Model file for the job. Use its own axes, mm. Face numbers are marked on the shaded views. A direction names the side the tool comes from. Round coordinates to 2 decimals unless told otherwise and drop trailing zeros. Loops run counter-clockwise (first coordinate to the right, second up) from the corner with the lowest first, then second, coordinate; pieces in that order, holes last. Notation, with made-up numbers: M -15,-28.75 L 18,-28.75 A27 cw 18,3.25 Z; hole C -24.5,43.25 d10. An arc over 180 degrees is marked long. Answer in a Markdown table with one row per item.
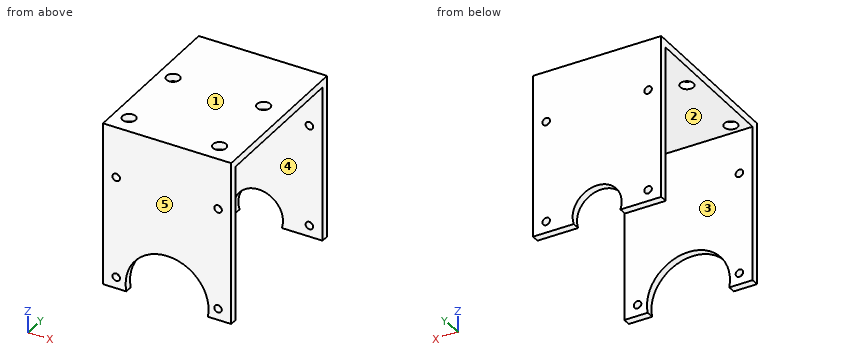
Autodesk Inventor part; units mm, degrees
ref_plane "YZ Plane" through (0, 0, 0) normal (1, 0, 0) x (0, 1, 0)
ref_plane "XZ Plane" through (0, 0, 0) normal (0, 1, 0) x (-1, 0, 0)
ref_plane "XY Plane" through (0, 0, 0) normal (0, 0, 1) x (1, 0, 0)
sketch "スケッチ1" plane through (0, 0, 0) normal (0, 1, 0) x (-1, 0, 0)
  line L0 (0, 0) -> (-34, 0)
  line L1 (-34, 0) -> (-34, -43.5)
  line L2 (-34, -43.5) -> (0, -43.5)
  line L3 (0, -43.5) -> (0, 0)
  dimension "d0" = 43.5
  dimension "d1" = 34
extrude "押し出し1" add sketch "スケッチ1" along normal blind 43.5
sketch "スケッチ2" plane through (34, 0, 0) normal (1, 0, 0) x (0, 0, -1)
  line L0 (2, 41.5) -> (52, 41.5)
  line L1 (52, 41.5) -> (52, 2)
  line L2 (52, 2) -> (2, 2)
  line L3 (2, 2) -> (2, 41.5)
  line L4 (0, 43.5) -> (43.5, 43.5)
  line L5 (0, 0) -> (0, 43.5)
  dimension "d4" = 2
  dimension "d5" = 2
  dimension "d6" = 39.5
  dimension "d7" = 50
extrude "押し出し2" cut sketch "スケッチ2" against normal blind 43.5
sketch "スケッチ3" plane through (0, 0, 0) normal (0, -1, 0) x (1, 0, 0)
  circle A0 centre (17, -41.5) radius 11
  line L0 (34, -43.5) -> (0, -43.5)
  line L1 (0, -43.5) -> (0, 0)
  point P0 (6.1833, -43.5)
  point P1 (27.8167, -43.5)
  dimension "d10" = 22
  dimension "d11" = 2
  dimension "d12" = 17
extrude "押し出し3" cut sketch "スケッチ3" against normal blind 2 contours A0 L0 picked at (20.7405, -37.2254)
sketch "スケッチ4" plane through (0, 43.5, 0) normal (0, 1, 0) x (1, 0, 0)
  circle A0 centre (17, 41.5) radius 6.5
  line L0 (34, 43.5) -> (0, 43.5)
  line L1 (0, 43.5) -> (0, 0)
  point P0 (23.1847, 43.5)
  point P1 (10.8153, 43.5)
  point P2 (0, 35.0774)
  dimension "d15" = 13
  dimension "d16" = 2
  dimension "d17" = 17
extrude "押し出し4" cut sketch "スケッチ4" against normal blind 2
sketch "スケッチ5" plane through (0, 43.5, 0) normal (0, 1, 0) x (1, 0, 0)
  line L0 (0, 0) -> (34, 0)
  line L1 (0, 43.5) -> (0, 0)
  line L2 (34, 0) -> (34, 43.5)
  point P0 (3.5, 13.5)
  point P1 (3.5, 40.5)
  point P2 (30.5, 40.5)
  point P3 (30.5, 13.5)
  dimension "d20" = 13.5
  dimension "d21" = 3.5
  dimension "d22" = 27
  dimension "d23" = 3.5
  dimension "d48" = 3.5
hole "穴1" at (3.5, 43.5, -13.5) at (3.5, 43.5, -40.5) at (30.5, 43.5, -40.5) at (30.5, 43.5, -13.5) direction (0, -1, 0) diameter 2 end through all
sketch "スケッチ6" plane through (0, 0, 0) normal (0, 0, 1) x (1, 0, 0)
  line L0 (0, 0) -> (34, 0)
  line L1 (0, 0) -> (0, 43.5)
  point P0 (4, 5)
  point P1 (4, 25)
  point P2 (28, 5)
  point P3 (28, 25)
  dimension "d31" = 5
  dimension "d32" = 4
  dimension "d35" = 20
  dimension "d38" = 24
hole "穴2" at (4, 5, 0) at (4, 25, 0) at (28, 5, 0) at (28, 25, 0) direction (0, 0, -1) diameter 3.5 end through all
properties part number "サーボモータ固定用"
1. Saw through at A-A (y = 25). Write the cut outline in (x, z).
Verdict:
| item | result |
|---|---|
| outline | M 0,-2 L 2.25,-2 L 2.25,0 L 0,0 Z; M 5.75,-2 L 26.25,-2 L 26.25,0 L 5.75,0 Z; M 29.75,-2 L 34,-2 L 34,0 L 29.75,0 Z |
2. Saw through at D-D (z = -37.5). Write the cut outline in (x, y).
Verdict:
| item | result |
|---|---|
| outline | M 0,0 L 6.75,0 L 6.75,2 L 0,2 Z; M 0,41.5 L 11.88,41.5 L 11.88,43.5 L 0,43.5 Z; M 22.12,41.5 L 34,41.5 L 34,43.5 L 22.12,43.5 Z; M 27.25,0 L 34,0 L 34,2 L 27.25,2 Z |
3. Tool access for the marked faces 4 and 5: list every direction of +Z, -Z, +X, -X, +Y, -Y with a clear straight run to the whole face (end or side of a thin tool).
Verdict:
| item | result |
|---|---|
| face 4 | -Z, +X, -X |
| face 5 | +Z, -Z, +X, -X, -Y |
4. Saw through at B-B (z = -24). Write the cut outline in (x, y).
Verdict:
| item | result |
|---|---|
| outline | M 0,0 L 34,0 L 34,2 L 0,2 Z; M 0,41.5 L 34,41.5 L 34,43.5 L 0,43.5 Z |
5. Pin check, flat tips, straight feed: pin 1 (10 mm diameter, centred on x = 4, y = 33.5, fed in from -Z); pin 2 (1.5 mm diameter, centred on x = 12, z = -34, fed in from -Y). Stop position of each tip, or through.
Verdict:
| item | result |
|---|---|
| pin 1 | stops at z = -2 |
| pin 2 | stops at y = 41.5 |
6. Wall check: probe 1 along X at (y, z) = (5, -1.05); probe 2 along Y at (x, z) = (2, -22.5); probe 3 along X at (y, z) = (0.8, -40.5). Give the ranges that are in metal, low to high.
Verdict:
| item | result |
|---|---|
| probe 1 | x = 0 to 2.25, 5.75 to 26.25, 29.75 to 34 |
| probe 2 | y = 0 to 2, 41.5 to 43.5 |
| probe 3 | x = 0 to 2.5, 4.5 to 6.05, 27.95 to 29.5, 31.5 to 34 |
7. Mould opens along Z. For the marked faces 1, 2 and 3 say: +Z half, -Z half, draft (parallel to the pull), parting line (faces both ways), or undercut.
Verdict:
| item | result |
|---|---|
| face 1 | +Z half |
| face 2 | -Z half |
| face 3 | draft |
8. Saw through at C-C (x = 30.5). Write the cut outline in (y, z), and give its area (3 significant figures).
Verdict:
| item | result |
|---|---|
| outline | M 0,-43.5 L 2,-43.5 L 2,-41.5 L 0,-41.5 Z; M 0,-39.5 L 2,-39.5 L 2,-14.5 L 0,-14.5 Z; M 0,-12.5 L 2,-12.5 L 2,-2 L 41.5,-2 L 41.5,-12.5 L 43.5,-12.5 L 43.5,0 L 0,0 Z; M 41.5,-43.5 L 43.5,-43.5 L 43.5,-41.5 L 41.5,-41.5 Z; M 41.5,-39.5 L 43.5,-39.5 L 43.5,-14.5 L 41.5,-14.5 Z |
| area | 237 mm² |
